Check sheet for the modelled part. Datum: model origin and axes. Units: mm. Face numbers are marked on the shaded views. A direction names the side the tool comes from. Coordinates: 2 decimals unless noted, no trailing zeros. Loops run counter-clockwise (first coordinate to the right, second up) from the corner with the lowest first, then second, coordinate; pieces in that order, holes last. Notation, with made-up numbers: (-3, -7) - (27, -7) arc R16 ccw to (27, 11) - close; hole circle Ø8 at (17, 8). An arc over 180 degrees is marked (long way). Write each question's results on one line, items separated by ' | '. Start each with the question number.
1. Draft check along Z on the marked faces 4, 5 and 6. Enter one of: released by +Z, released by -Z, zero draft, split by the parting line, or undercut.
2. Cross-section at C-C (z = 2). Record the cut outline in (x, y), and give its area (3 significant figures).
3. Cross-section at A-A (x = 0). Record the cut outline in (y, z), and give its area (3 significant figures).
4. Tool access check on the marked faces 1, 2 and 3. Record the directions out of +Z, -Z, +X, -X, +Y, -Y that give a thin tool (end or side, any length) a straight path to the whole face; none if there is none.
5. Thickness scan on line 1 (X direction, y = -8, z = 42.5); line 2 (X direction, y = -18.25, z = -37); line 3 (Z direction, x = -0.5, y = -3). Record the ranges inside material, lowest first. Write a range as [from, to].
6. Cross-section at B-B (z = -39.5). Record the cut outline in (x, y).
7. Gauge pin test, flat ends, axial feed: P1, Ø1, axis at y = -18.5, z = -20, coming from the +X side; P2, Ø1, axis at x = -19, z = -4, coming from the +Y side; P3, Ø7, axis at y = -7, z = 46.5, coming from the +X side; P4, Ø3, axis at y = -16, z = 39, coming from the +X side. Record the tip position at first contact, or that the pin passes through.
```python
from build123d import *

# Parameters (mm, degrees)
F0_R     = 10.769263
F1_DEPTH = 25


with BuildPart() as f1:
    # F0 (on Front) → F1 (new body)
    with BuildSketch(Plane.XZ):
        with BuildLine():
            ThreePointArc((41.013222, -1.92807), (41.047192, -0.964301), (41.058517, 0))
            ThreePointArc((41.058517, 0), (40.631678, 5.904962), (39.360035, 11.68715))
            ThreePointArc((39.360035, 11.68715), (38.390381, 14.559551), (37.211423, 17.352574))
            ThreePointArc((37.211423, 17.352574), (33.790497, 23.323896), (29.420291, 28.639978))
            ThreePointArc((29.420291, 28.639978), (27.226833, 30.732742), (24.884936, 32.657952))
            ThreePointArc((24.884936, 32.657952), (19.080844, 36.355512), (12.740712, 39.031732))
            ThreePointArc((12.740712, 39.031732), (9.825946, 39.865431), (6.85761, 40.481786))
            ThreePointArc((6.85761, 40.481786), (0, 41.058517), (-6.85761, 40.481786))
            ThreePointArc((-6.85761, 40.481786), (-9.825946, 39.865431), (-12.740712, 39.031732))
            ThreePointArc((-12.740712, 39.031732), (-19.080844, 36.355512), (-24.884936, 32.657952))
            ThreePointArc((-24.884936, 32.657952), (-27.226833, 30.732742), (-29.420291, 28.639978))
            ThreePointArc((-29.420291, 28.639978), (-33.790497, 23.323896), (-37.211423, 17.352574))
            ThreePointArc((-37.211423, 17.352574), (-38.390381, 14.559551), (-39.360035, 11.68715))
            ThreePointArc((-39.360035, 11.68715), (-40.759155, 4.949057), (-41.013222, -1.92807))
            ThreePointArc((-41.013222, -1.92807), (-40.759155, -4.949057), (-40.28287, -7.943063))
            ThreePointArc((-40.28287, -7.943063), (-38.390381, -14.559551), (-35.419386, -20.767016))
            ThreePointArc((-35.419386, -20.767016), (-33.790497, -23.323896), (-31.977384, -25.753616))
            ThreePointArc((-31.977384, -25.753616), (-27.226833, -30.732742), (-21.711395, -34.848489))
            ThreePointArc((-21.711395, -34.848489), (-19.080844, -36.355512), (-16.346266, -37.664326))
            ThreePointArc((-16.346266, -37.664326), (-9.825946, -39.865431), (-3.029586, -40.946593))
            ThreePointArc((-3.029586, -40.946593), (0, -41.058517), (3.029586, -40.946593))
            ThreePointArc((3.029586, -40.946593), (9.825946, -39.865431), (16.346266, -37.664326))
            ThreePointArc((16.346266, -37.664326), (19.080844, -36.355512), (21.711395, -34.848489))
            ThreePointArc((21.711395, -34.848489), (27.226833, -30.732742), (31.977384, -25.753616))
            ThreePointArc((31.977384, -25.753616), (33.790497, -23.323896), (35.419386, -20.767016))
            ThreePointArc((35.419386, -20.767016), (38.390381, -14.559551), (40.28287, -7.943063))
            ThreePointArc((40.28287, -7.943063), (40.759155, -4.949057), (41.013222, -1.92807))
        make_face()
        Circle(F0_R, mode=Mode.SUBTRACT)
        with BuildLine():
            ThreePointArc((39.360035, 11.68715), (40.631678, 5.904962), (41.058517, 0))
            ThreePointArc((41.058517, 0), (41.047192, -0.964301), (41.013222, -1.92807))
            Line((41.013222, -1.92807), (49.50533, -0.896941))
            Line((49.50533, -0.896941), (47.852143, 12.718279))
            Line((47.852143, 12.718279), (39.360035, 11.68715))
        make_face()
        with BuildLine():
            ThreePointArc((29.420291, 28.639978), (33.790497, 23.323896), (37.211423, 17.352574))
            Line((37.211423, 17.352574), (44.251622, 22.212072))
            Line((44.251622, 22.212072), (36.460489, 33.499476))
            Line((36.460489, 33.499476), (29.420291, 28.639978))
        make_face()
        with BuildLine():
            Line((48.281447, -10.976523), (40.28287, -7.943063))
            ThreePointArc((40.28287, -7.943063), (38.390381, -14.559551), (35.419386, -20.767016))
            Line((35.419386, -20.767016), (43.417963, -23.800476))
            Line((43.417963, -23.800476), (48.281447, -10.976523))
        make_face()
        with BuildLine():
            ThreePointArc((12.740712, 39.031732), (19.080844, 36.355512), (24.884936, 32.657952))
            Line((24.884936, 32.657952), (28.860401, 40.232567))
            Line((28.860401, 40.232567), (16.716177, 46.606347))
            Line((16.716177, 46.606347), (12.740712, 39.031732))
        make_face()
        with BuildLine():
            Line((37.650053, -32.156736), (31.977384, -25.753616))
            ThreePointArc((31.977384, -25.753616), (27.226833, -30.732742), (21.711395, -34.848489))
            Line((21.711395, -34.848489), (27.384064, -41.251608))
            Line((27.384064, -41.251608), (37.650053, -32.156736))
        make_face()
        with BuildLine():
            ThreePointArc((-6.85761, 40.481786), (0, 41.058517), (6.85761, 40.481786))
            Line((6.85761, 40.481786), (6.85761, 49.036266))
            Line((6.85761, 49.036266), (-6.85761, 49.036266))
            Line((-6.85761, 49.036266), (-6.85761, 40.481786))
        make_face()
        with BuildLine():
            Line((18.393487, -45.970228), (16.346266, -37.664326))
            ThreePointArc((16.346266, -37.664326), (9.825946, -39.865431), (3.029586, -40.946593))
            Line((3.029586, -40.946593), (5.076807, -49.252495))
            Line((5.076807, -49.252495), (18.393487, -45.970228))
        make_face()
        with BuildLine():
            ThreePointArc((-24.884936, 32.657952), (-19.080844, 36.355512), (-12.740712, 39.031732))
            Line((-12.740712, 39.031732), (-16.716177, 46.606347))
            Line((-16.716177, 46.606347), (-28.860401, 40.232567))
            Line((-28.860401, 40.232567), (-24.884936, 32.657952))
        make_face()
        with BuildLine():
            Line((-5.076807, -49.252495), (-3.029586, -40.946593))
            ThreePointArc((-3.029586, -40.946593), (-9.825946, -39.865431), (-16.346266, -37.664326))
            Line((-16.346266, -37.664326), (-18.393487, -45.970228))
            Line((-18.393487, -45.970228), (-5.076807, -49.252495))
        make_face()
        with BuildLine():
            ThreePointArc((-37.211423, 17.352574), (-33.790497, 23.323896), (-29.420291, 28.639978))
            Line((-29.420291, 28.639978), (-36.460489, 33.499476))
            Line((-36.460489, 33.499476), (-44.251622, 22.212072))
            Line((-44.251622, 22.212072), (-37.211423, 17.352574))
        make_face()
        with BuildLine():
            Line((-27.384064, -41.251608), (-21.711395, -34.848489))
            ThreePointArc((-21.711395, -34.848489), (-27.226833, -30.732742), (-31.977384, -25.753616))
            Line((-31.977384, -25.753616), (-37.650053, -32.156736))
            Line((-37.650053, -32.156736), (-27.384064, -41.251608))
        make_face()
        with BuildLine():
            ThreePointArc((-41.013222, -1.92807), (-40.759155, 4.949057), (-39.360035, 11.68715))
            Line((-39.360035, 11.68715), (-47.852143, 12.718279))
            Line((-47.852143, 12.718279), (-49.50533, -0.896941))
            Line((-49.50533, -0.896941), (-41.013222, -1.92807))
        make_face()
        with BuildLine():
            Line((-43.417963, -23.800476), (-35.419386, -20.767016))
            ThreePointArc((-35.419386, -20.767016), (-38.390381, -14.559551), (-40.28287, -7.943063))
            Line((-40.28287, -7.943063), (-48.281447, -10.976523))
            Line((-48.281447, -10.976523), (-43.417963, -23.800476))
        make_face()
    extrude(amount=F1_DEPTH)


solid = f1.part
```
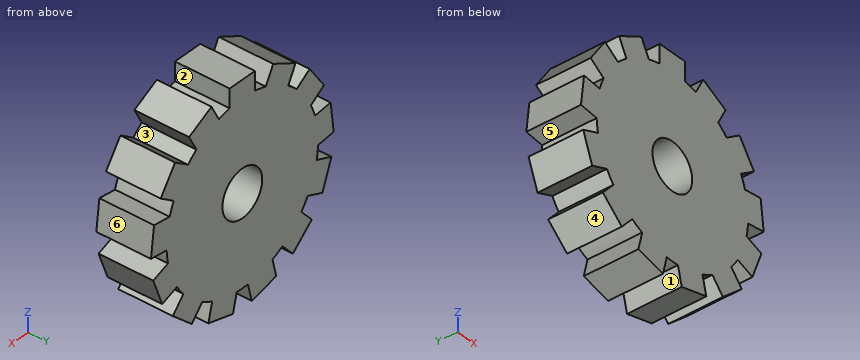
Established:
1) face 4: released by -Z | face 5: undercut | face 6: released by +Z
2) outline: (-49.15, -25) - (-10.58, -25) - (-10.58, 0) - (-49.15, 0) - close; (10.58, -25) - (49.15, -25) - (49.15, 0) - (10.58, 0) - close | area: 1,930 mm^2
3) outline: (-25, -41.06) - (0, -41.06) - (0, -10.77) - (-25, -10.77) - close; (-25, 10.77) - (0, 10.77) - (0, 49.04) - (-25, 49.04) - close | area: 1,710 mm^2
4) face 1: -Z, +Y, -Y | face 2: +Z, +Y, -Y | face 3: +Y, -Y
5) line 1: [-24.54, -14.56], [-6.86, 6.86], [14.56, 24.54] | line 2: [-32.18, -23.62], [-17.8, 17.8], [23.62, 32.18] | line 3: [-41.06, -10.76], [10.76, 49.04]
6) outline: (-29.36, -25) - (-25.83, -25) - (-25.83, 0) - (-29.36, 0) - close; (-16.8, -25) - (16.8, -25) - (16.8, 0) - (-16.8, 0) - close; (25.83, -25) - (29.36, -25) - (29.36, 0) - (25.83, 0) - close
7) P1: x = 45.05 | P2: y = 0 | P3: x = 23.59 | P4: x = 28.86
